Read the model definition and answer for the solid it produces. Units are mm, in the model's axes. Face numbers are marked on the shaded views. Coordinates: 2 decimals unless noted, no trailing zeros. Loops run counter-clockwise (first coordinate to the right, second up) from the corner with the lowest first, then second, coordinate; pieces in that order, holes last. Notation, with made-up numbers: (73, 85.5) -> (118, 85.5) arc R25 cw to (118, 102.5) -> close; hole circle Ø10 at (-21.75, 20). An arc over 180 degrees is marked (long way). Answer as a JSON object with one key per item and string values. Group by question number.
1) Determine the mould class of the marked faces 1, 2 and 3 for opening direction X: released by +X, released by -X, zero draft, split by the parting line, or undercut.
2) Consider probe 1 along Z at (x, y) = (-20.5, 164); probe 2 along X at (y, z) = (96, -117.5); probe 3 along Z at (x, y) = (-3.5, 209). Determine where each line is inside the solid, lowest interval first. Write a range as [from, to].
3) Flat-ended cylindrical pins translate along their axes: P1, Ø6, axis at y = 10, z = -74.41, coming from the +X side; P2, Ø2, axis at x = -23, y = 126, coming from the +Z side; P3, Ø6, axis at y = 56, z = -150.5, coming from the -X side. Find the tip coordinate at first contact, or state that the pin passes through.
4) Section A-A, the plane x = -17.5 is taken. Give the vertices of the cut face in (y, z), plus the area to 3 significant figures.
5) Section D-D, the plane y = 186.5 is taken. Give the vertices of the cut face in (x, z), plus the area to 3 significant figures.
6) Section B-B, the plane y = 144.5 is taken. Give the vertices of the cut face in (x, z), plus the area to 3 significant figures.
7) Section C-C, the plane z = -166 is taken. Give the vertices of the cut face in (x, y).
from build123d import *

# Parameters (mm, degrees)
F1_DEPTH = 320
F2_R     = 5
F3_DEPTH = 1.2
F4_R     = 5
F6_DEPTH = 1.2
F7_R     = 2.5
F8_DEPTH = 1.2


with BuildPart() as f1:
    # F0 (on Front) → F1 (new body)
    with BuildSketch(Plane.XZ):
        with BuildLine():
            Line((1.2, 0), (0, 0))
            Line((0, 0), (0, -207))
            ThreePointArc((0, -207), (-1.464466, -210.535534), (-5, -212))
            Line((-5, -212), (-30, -212))
            Line((-30, -212), (-30, -213.2))
            Line((-30, -213.2), (-5, -213.2))
            ThreePointArc((-5, -213.2), (-0.615938, -211.384062), (1.2, -207))
            Line((1.2, -207), (1.2, 0))
        make_face()
    extrude(amount=-F1_DEPTH)

    # F2 (on face) → F3 (cut, through all)
    with BuildSketch(Plane.XY.offset(-212)):
        with Locations((-17.5, 305)):
            Circle(F2_R)
        with Locations((-17.5, 15)):
            Circle(F2_R)
    extrude(amount=-F3_DEPTH, mode=Mode.SUBTRACT)

    # F4
    f4_edges = [f1.edges().sort_by_distance(p)[0] for p in [
        (-30, 320, -212.6),
        (-30, 0, -212.6),
    ]]
    fillet(f4_edges, radius=F4_R)

    # F5 (on face) → F6 (cut, through all)
    with BuildSketch(Plane(origin=(0, 0, 0), x_dir=(0, -1, 0), z_dir=(-1, 0, 0))):
        Polygon((0, 0), (-320, 0), (-320, -35), (0, -55), align=None)
    extrude(amount=-F6_DEPTH, mode=Mode.SUBTRACT)

    # F7 (on face) → F8 (cut, through all)
    with BuildSketch(Plane.YZ.offset(1.2)):
        with Locations((10, -74.414024)):
            Circle(F7_R)
        with Locations((159.707887, -65.057282)):
            Circle(F7_R)
        with Locations((309.415774, -55.700539)):
            Circle(F7_R)
    extrude(amount=-F8_DEPTH, mode=Mode.SUBTRACT)


solid = f1.part
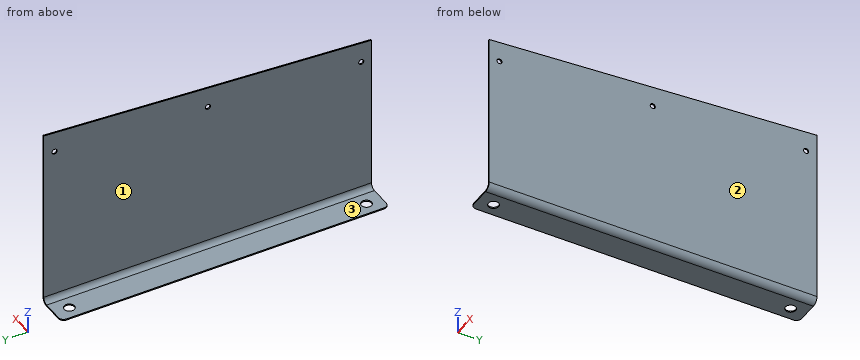
Determined:
{
 "1": {"face 1": "released by -X", "face 2": "released by +X", "face 3": "zero draft"},
 "2": {"probe 1": "[-213.2, -212]", "probe 2": "[0, 1.2]", "probe 3": "[-213.02, -211.77]"},
 "3": {"P1": "x = 1.2", "P2": "z = -212", "P3": "x = 0"},
 "4": {"outline": "(0, -213.2) -> (10, -213.2) -> (10, -212) -> (0, -212) -> close; (20, -213.2) -> (300, -213.2) -> (300, -212) -> (20, -212) -> close; (310, -213.2) -> (320, -213.2) -> (320, -212) -> (310, -212) -> close", "area": "360 mm²"},
 "5": {"outline": "(-30, -213.2) -> (-5, -213.2) arc R6.2 ccw to (1.2, -207) -> (1.2, -43.34) -> (0, -43.34) -> (0, -207) arc R5 cw to (-5, -212) -> (-30, -212) -> close", "area": "237 mm²"},
 "6": {"outline": "(-30, -213.2) -> (-5, -213.2) arc R6.2 ccw to (1.2, -207) -> (1.2, -45.97) -> (0, -45.97) -> (0, -207) arc R5 cw to (-5, -212) -> (-30, -212) -> close", "area": "234 mm²"},
 "7": {"outline": "(0, 0) -> (1.2, 0) -> (1.2, 320) -> (0, 320) -> close"}
}
